Here's how the part is built. I have some questions about the finished solid (model axes, mm). Face numbers are marked on the shaded views. A direction names the side the tool comes from. Round coordinates to 2 decimals unless told otherwise and drop trailing zeros. Loops run counter-clockwise (first coordinate to the right, second up) from the corner with the lowest first, then second, coordinate; pieces in that order, holes last. Notation, with made-up numbers: (25, -30) -> (53, -30) arc R8 cw to (53, -20) -> close; hole circle Ø8 at (39.5, 4). An arc over 180 degrees is marked (long way). One line per item, written item: value. Start each with the question number.
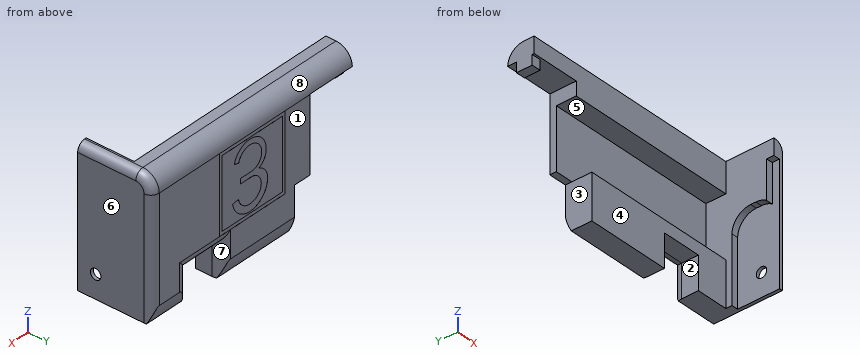
Autodesk Inventor part; units mm, degrees
ref_plane "作業平面1" through (-54.9, 2, -8) normal (1, 0, 0) x (0, 1, 0)
ref_plane "作業平面2" through (-69.8, 2, -8) normal (-1, 0, 0) x (0, 0, 1)
ref_plane "YZ Plane" through (0, 0, 0) normal (1, 0, 0) x (0, 1, 0)
sketch "スケッチ1" plane through (0, 0, 0) normal (1, 0, 0) x (0, 1, 0)
  line L0 (0, 0) -> (22.8, 0)
  line L1 (22.8, 0) -> (22.8, 41.3)
  line L2 (22.8, 41.3) -> (0, 41.3)
  line L3 (0, 41.3) -> (0, 0)
  arc A0 (2, -7.1682) -> (22.8, 4.7165) centre (7.1, 8.05) ccw
  line L4 (22.8, 36.2) -> (22.8, 4.7165)
  line L5 (22.8, 36.2) -> (12.6, 36.2)
  line L6 (12.6, 36.2) -> (12.6, 28.2)
  line L7 (14.2, 28.2) -> (12.6, 28.2)
  line L8 (14.2, 28.2) -> (14.2, 32.2)
  line L9 (14.2, 32.2) -> (20.8, 32.2)
  line L10 (20.8, 32.2) -> (20.8, 8.3)
  line L11 (14.2, 8.3) -> (20.8, 8.3)
  line L12 (14.2, 4.7954) -> (14.2, 8.3)
  line L13 (14.2, 0) -> (14.2, 4.7954)
  line L14 (2, 0) -> (14.2, 0)
  line L15 (2, 0) -> (2, -7.1682)
  line L16 (12.6, 42.3) -> (14.6, 42.3)
  dimension "d2" = 1
extrude "押し出し1" add sketch "スケッチ1" along normal blind 1 contours L3 L2 L1 L5 L6 L7 L8 L9 L10 L11 L12 L13 L0 | L13 L12 L11 L10 L9 L8 L7 L6 L5 L1 A0 L0 | A0 L1 L0
sketch "スケッチ2" plane through (0, 0, 0) normal (-1, 0, 0) x (0, 0, 1)
  line L0 (24.3426, 2) -> (36.2, 2)
  line L1 (36.2, 0) -> (36.2, 2)
  arc A0 (25.6, 7.1) -> (20.1, 12.6) centre (20.1, 7.1) ccw
  line L2 (25.6, 7.1) -> (25.6, 5.5)
  arc A1 (24.3426, 2) -> (25.6, 5.5) centre (20.1, 5.5) ccw
  line L3 (0, 12.6) -> (20.1, 12.6)
  line L4 (0, 22.8) -> (41.3, 22.8)
  line L5 (0, 0) -> (0, 22.8)
  line L6 (41.3, 0) -> (0, 0)
  line L7 (41.3, 22.8) -> (41.3, 0)
  line L8 (0, 12.8) -> (20.1, 12.8)
  arc A2 (25.8, 7.1) -> (20.1, 12.8) centre (20.1, 7.1) ccw
  arc A3 (24.7476, 2.2) -> (25.8, 5.5) centre (20.1, 5.5) ccw
  line L9 (25.8, 5.5) -> (25.8, 7.1)
  line L10 (24.7476, 2.2) -> (36.4, 2.2)
  line L11 (36.4, 2.2) -> (36.4, 0)
  line L12 (41.3, 0) -> (0, 0)
  line L13 (0, 0) -> (0, 22.8)
extrude "押し出し2" add sketch "スケッチ2" along normal blind 2 contours L11 L10 A3 L9 A2 L8 L5 L4 L7 L6
sketch "スケッチ3" plane through (-2, 0, 0) normal (-1, 0, 0) x (0, 0, 1)
  line L0 (28.2, 12.6) -> (50.1, 12.6)
  line L1 (0, 14.2) -> (4.55, 14.2)
  line L2 (41.3, 0) -> (41.3, 22.8)
  line L3 (41.3, 22.8) -> (0, 22.8)
  line L4 (0, 22.8) -> (0, 12.8)
  line L5 (0, 12.8) -> (20.1, 12.8)
  arc A0 (25.8, 7.1) -> (20.1, 12.8) centre (20.1, 7.1) ccw
  line L6 (25.8, 7.1) -> (25.8, 5.5)
  arc A1 (24.7476, 2.2) -> (25.8, 5.5) centre (20.1, 5.5) ccw
  line L7 (24.7476, 2.2) -> (36.4, 2.2)
  line L8 (36.4, 2.2) -> (36.4, 0)
  line L9 (36.4, 0) -> (41.3, 0)
  line L10 (41.3, 0) -> (41.3, 22.8)
  line L11 (0, 14.7) -> (41.3, 14.7)
  point P0 (0, 0)
  dimension "d9" = 0.5
extrude "押し出し3" add sketch "スケッチ3" along normal blind 47.4 contours L11 L4 L3 L2
sketch "スケッチ4" plane through (-49.4, 0, 0) normal (-1, 0, 0) x (0, 0, 1)
  line L0 (11.075, 12.3395) -> (13.693, 16.874)
  line L1 (13.693, 16.874) -> (13.693, 22.8)
  line L2 (41.3, 22.8) -> (0, 22.8)
  line L3 (0, 22.8) -> (0, 14.7)
  line L4 (0, 14.7) -> (41.3, 14.7)
  line L5 (41.3, 14.7) -> (41.3, 22.8)
  line L6 (41.3, 22.8) -> (0, 22.8)
  arc A0 (4.7165, 22.8) -> (-7.1682, 2) centre (8.05, 7.1) ccw
  line L7 (36.2, 22.8) -> (4.7165, 22.8)
  line L8 (36.2, 22.8) -> (36.2, 12.6)
  line L9 (36.2, 12.6) -> (28.2, 12.6)
  line L10 (28.2, 14.2) -> (28.2, 12.6)
  line L11 (28.2, 14.2) -> (32.2, 14.2)
  line L12 (32.2, 14.2) -> (32.2, 20.8)
  line L13 (32.2, 20.8) -> (8.3, 20.8)
  line L14 (8.3, 14.2) -> (8.3, 20.8)
  line L15 (4.7954, 14.2) -> (8.3, 14.2)
  line L16 (0, 14.2) -> (4.7954, 14.2)
  line L17 (0, 2) -> (0, 14.2)
  line L18 (0, 2) -> (-7.1682, 2)
  point P0 (0, 0)
  point P1 (13.693, 20.8)
  point P2 (32.2, 14.7)
ref_plane "作業平面1" through (-54.9, 2, -8) normal (1, 0, 0) x (0, 1, 0)
extrude "押し出し4" add sketch "スケッチ4" along normal up to surface (5.5 mm away) contours L12 L13 L1 L2 L8 L4 | L8 L2 L5 L4
sketch "スケッチ5" plane through (-54.9, 14.7, 41.3) normal (-1, 0, 0) x (0, 0, 1)
  line L0 (-27.607, 6.1) -> (-9.1, 6.1)
  line L1 (-9.1, 6.1) -> (-9.1, 0)
  line L2 (-9.1, 0) -> (0, 0)
  line L3 (0, 0) -> (0, 8.1)
  line L4 (0, 8.1) -> (-27.607, 8.1)
  line L5 (-27.607, 8.1) -> (-27.607, 6.1)
  line L6 (-5.1, -12.7) -> (-5.1, 0.5)
  line L7 (0, 0) -> (-41.3, 0)
  line L8 (-4.9, 0) -> (-4.9, 8.1)
  point P0 (-41.3, -14.7)
  point P1 (-4.9, 0)
  dimension "d14" = 0.2
ref_plane "作業平面2" through (-69.8, 2, -8) normal (-1, 0, 0) x (0, 0, 1)
extrude "押し出し5" add sketch "スケッチ5" along normal up to surface (14.9 mm away) contours L4 L3 L2 L8
sketch "スケッチ6" plane through (-49.4, 0, 0) normal (-1, 0, 0) x (0, 0, 1)
  line L0 (13.693, 20.8) -> (13.693, 22.8)
  line L1 (13.693, 22.8) -> (0, 22.8)
  line L2 (0, 22.8) -> (0, 14.7)
  line L3 (0, 14.7) -> (32.2, 14.7)
  line L4 (32.2, 14.7) -> (32.2, 20.8)
  line L5 (32.2, 20.8) -> (13.693, 20.8)
  line L6 (13.693, 20.8) -> (13.693, 14.7)
  point P0 (0, 0)
extrude "押し出し6" cut sketch "スケッチ6" against normal up to surface (47.4 mm away) contours L5 L4 L3 L6
fillet "フィレット1" radius 5 1 edges at (-34.4, 22.8, 41.3)
fillet "フィレット2" radius 2.5 3 edges at (1, 22.8, 18.15) (1, 21.3355, 39.8355) (1, 8.9, 41.3)
sketch "スケッチ7" plane through (-49.4, 0, 0) normal (-1, 0, 0) x (0, 0, 1)
  arc A0 (4.7165, 22.8) -> (-7.1682, 2) centre (8.05, 7.1) ccw
  line L0 (13.693, 22.8) -> (0, 22.8)
  arc A1 (4.7165, 22.8) -> (-7.1682, 2) centre (8.05, 7.1) ccw
  line L1 (0, 22.8) -> (0, 14.7)
  point P0 (0, 0)
  point P1 (0, 20.9852)
extrude "押し出し7" cut sketch "スケッチ7" against normal through all
sketch "スケッチ8" plane through (0, 0, 0) normal (0, 0, -1) x (-1, 0, 0)
  line L0 (23.7, 13.1) -> (23.7, 1.1)
  line L1 (2, 14.7) -> (49.4, 14.7)
  line L2 (1.5, 22.8) -> (49.4, 22.8)
  line L3 (2, 14.7) -> (69.8, 14.7)
  line L4 (23.7, 14.7) -> (11.7, 14.7)
  line L5 (11.7, 14.7) -> (11.7, 22.8)
  line L6 (11.7, 22.8) -> (23.7, 22.8)
  line L7 (23.7, 22.8) -> (23.7, 14.7)
  point P0 (0, 0)
  point P1 (11.7, 14.7)
  dimension "d23" = 12
extrude "押し出し8" cut sketch "スケッチ8" against normal blind 10
fillet "フィレット3" radius 3 3 edges at (-23.7, 22.8, 7.3582) (-11.7, 22.8, 7.3582) (-17.7, 22.8, 10)
sketch "スケッチ9" plane through (-69.8, 14.7, 36.4) normal (-1, 0, 0) x (0, 0, 1)
  line L0 (-0.2, 0.5) -> (-3.2, 0.5)
  line L1 (-0.2, 5.5) -> (-0.2, 0.5)
  line L2 (-3.2, 5.5) -> (-0.2, 5.5)
  line L3 (-3.2, 0.5) -> (-3.2, 5.5)
  line L4 (-3, 5.4) -> (0, 5.4)
  line L5 (0, 5.4) -> (0, 0.6)
  line L6 (0, 0.6) -> (-3, 0.6)
  line L7 (-3, 0.6) -> (-3, 5.4)
  arc A0 (4.9, 3.1) -> (0, 8.099) centre (-0.1, 3.1) ccw
  line L8 (0, 0) -> (0, 8.099)
  line L9 (4.9, 0) -> (0, 0)
  line L10 (4.9, 3.1) -> (4.9, 0)
  line L11 (0, 0) -> (0, 8.099)
  point P0 (-36.4, -14.7)
  point P1 (-0.2, 3)
  point P2 (-3, 3)
  dimension "d27" = 4.8
extrude "押し出し9" add sketch "スケッチ9" against normal blind 2.8 contours L6 L7 L4 L1 | L1 L4 L5 L6
sketch "スケッチ10" plane through (1, 0, 0) normal (1, 0, 0) x (0, 0, -1)
  circle A0 centre (-7.05, 5.504) radius 1.6
  arc A1 (-4.65, 5.508) -> (-6.95, 8) centre (-7.15, 5.508) ccw
  arc A2 (-6.95, 8) -> (-9.45, 5.5) centre (-6.95, 5.5) ccw
  line L0 (-7.15, 5.508) -> (-6.95, 5.5)
  point P0 (0, 0)
  dimension "d30" = 3.2
extrude "押し出し10" cut sketch "スケッチ10" against normal through all
sketch "スケッチ11" plane through (-54.9, 22.8, 13.693) normal (0, 1, 0) x (1, 0, 0)
  line L0 (53.4, -22.607) -> (0, -22.607)
  line L1 (32.15, -22.607) -> (8.85, -22.607)
  line L2 (8.85, -22.607) -> (8.85, 0.693)
  line L3 (8.85, 0.693) -> (32.15, 0.693)
  line L4 (32.15, 0.693) -> (32.15, -22.607)
  line L5 (28.2, 0.693) -> (46.2, 0.693)
  line L6 (20.5, -22.607) -> (20.5, -17.7274)
  line L7 (55.9, -22.607) -> (55.9, 13.693)
  line L8 (-14.9, -27.607) -> (-14.9, -22.707)
  line L9 (55.9, -22.607) -> (55.9, 7.9184)
  line L10 (-14.9, -27.607) -> (-14.9, -22.707)
  line L11 (-14.9, -27.607) -> (-14.9, -22.707)
  line L12 (10.35, -0.807) -> (30.65, -0.807)
  line L13 (30.65, -0.807) -> (30.65, -21.107)
  line L14 (30.65, -21.107) -> (10.35, -21.107)
  line L15 (10.35, -21.107) -> (10.35, -0.807)
  line L16 (9.85, -0.307) -> (31.15, -0.307)
  line L17 (31.15, -0.307) -> (31.15, -21.607)
  line L18 (31.15, -21.607) -> (9.85, -21.607)
  line L19 (9.85, -21.607) -> (9.85, -0.307)
  line L20 (-14.2639, 8.2606) -> (-10.5139, 8.2606)
  circle A0 centre (21.3, -7.057) radius 6.25
  circle A1 centre (21.3, -15.357) radius 5.75
  circle A2 centre (21.3, -7.057) radius 4.15
  circle A3 centre (21.3, -15.357) radius 4.15
  line L21 (24.6204, -10.2528) -> (18.6525, -10.2528)
  line L22 (18.6525, -10.2528) -> (18.6525, -11.7867)
  line L23 (18.6525, -11.7867) -> (24.6204, -11.7867)
  line L24 (24.6204, -11.7867) -> (24.6204, -10.2528)
  arc A4 (15.053, -6.8649) -> (21.3, -11.207) centre (19.5885, -7.0044) ccw
  arc A5 (21.3, -11.207) -> (15.55, -15.3584) centre (19.9229, -15.3573) ccw
  arc A6 (20.7203, -11.7867) -> (17.15, -15.357) centre (20.7203, -15.357) ccw
  arc A7 (18.3285, -4.16) -> (20.8976, -10.2528) centre (20.8976, -6.6647) ccw
  line L25 (21.3, -15.357) -> (26.8541, -16.8452)
  line L26 (21.3, -7.057) -> (27.455, -5.9717)
  point P0 (54.9, 13.693)
  point P1 (20.5, 14.3955)
  point P2 (30.65, -10.957)
  point P3 (31.15, -10.957)
  point P4 (20.5, -0.807)
  point P5 (20.5, -0.307)
  point P6 (20.5, 3.8955)
  point P7 (18.6525, -11.0197)
  point P8 (32.15, -10.957)
  point P9 (20.5, -21.607)
  point P10 (25.387, -6.3363)
  point P11 (18.2184, -11.3303)
  point P12 (25.3086, -16.4311)
  point P13 (8.85, -22.607)
  dimension "d33" = 35.4
  dimension "d34" = 35.4
  dimension "d35" = 23.3
  dimension "d36" = 23.3
  dimension "d40" = 0.5
  dimension "d49" = 1
  dimension "d51" = 11.5
  dimension "d52" = 12.5
  dimension "d53" = 0.8
  dimension "d54" = 80
  dimension "d55" = 75
extrude "押し出し11" cut sketch "スケッチ11" against normal blind 0.01 contours L0 L2 L3 L4 | A1 A5 A0 A3 L6 | L6 A3 L25 A1 | A3 A0 A6 | A5 A4 L22 L23 A3 A0 | A0 L26 A2 A1 A4 | A3 L23 A6 A0 | A1 L22 A5 A4 | A5 L22 A4 | L23 L22 A4 A3 | A3 A4 L23 | A2 A7 A1 | L21 A2 A5 | A1 A7 L21 | A2 A5 L22 | L22 A5 A2 A3 A4 | L24 L23 A3 A2 A1 | A1 L21 L24 | A3 A4 | A5 A2 picked at (17.7249, -13.3851) picked at (19.4043, -11.9435) picked at (18.4353, -9.7598) picked at (19.6416, -10.192)
equation "\"d33\" = d34"
equation "\"d36\" = d35"
equation "\"d4\" = d3"
equation "\"d5\" = d4"
equation "\"d6\" = d5"
properties part number "hand_finger_cover_3"
Q1. I want a section at D-D on x = -16. Please give me the cut outline in (y, z), plus the area to 3 significant figures.
Q2. I want a section at A-A on z = 7.05. Please give me the cut outline in (x, y).
Q3. Which directions (+Z, -Z, +X, -X, +Y, -Y) give clear straight access to the entire face, cutting with the end or side of a thin tool? Please do the marked faces 1, 2, 3, 4 and 5.
Q4. I want a section at B-B on x = -5.5. Please give me the cut outline in (y, z), plus the area to 3 significant figures.
Q5. If we mould it in two halves opening along X, with no side actions, what happens to the marked faces 6, 7 and 8? For each: released by +X, released by -X, zero draft, split by the parting line, or undercut.
Q6. Will these pins go through, and if not, where does the flat tip stop? P1, Ø2.5, axis at y = 5.504, z = 7.05, coming from the -X side; P2, Ø2, axis at x = -68, y = 18, coming from the -Z side; P3, Ø5, axis at x = -50, z = 23.5, coming from the -Y side; P4, Ø4, axis at x = -16, y = 18.5, coming from the -Z side.
Q7. If I drill on line 1 along Z through (x, y) = (-36, 16); line 2 along Y through (x, z) = (-48, 36.5); line 3 along X through (y, z) = (18.25, 7), over which ranges is the centre line in solid material (lowest first)?
Answers below:
1. outline: (14.7, 10) -> (19.8, 10) arc R3 ccw to (22.8, 13) -> (22.8, 36.3) arc R5 ccw to (17.8, 41.3) -> (14.7, 41.3) -> (14.7, 32.2) -> (20.8, 32.2) -> (20.8, 13.69) -> (14.7, 13.69) -> close
1. area: 133 mm^2
2. outline: (-49.4, 14.7) -> (-23.7, 14.7) -> (-23.7, 19.8) arc R3 ccw to (-26.7, 22.8) -> (-49.4, 22.8) -> close; (-11.7, 14.7) -> (-2, 14.7) -> (-2, 12.8) -> (0, 12.8) -> (0, 7.1) -> (1, 7.1) -> (1, 20.3) arc R2.5 ccw to (-1.5, 22.8) -> (-8.7, 22.8) arc R3 ccw to (-11.7, 19.8) -> close; (0, 0) -> (1, 0) -> (1, 3.9) -> (0, 3.9) -> close
3. face 1: +Z, -Z, +X, -X, +Y
3. face 2: -Z, +Y, -Y
3. face 3: -Z, -X, +Y, -Y
3. face 4: +Z, -Z, -X, -Y
3. face 5: -X, -Y
4. outline: (14.7, 0) -> (20.99, 0) arc R16.05 ccw to (22.8, 4.72) -> (22.8, 36.3) arc R5 ccw to (17.8, 41.3) -> (14.7, 41.3) -> (14.7, 32.2) -> (20.8, 32.2) -> (20.8, 13.69) -> (14.7, 13.69) -> close
4. area: 213 mm^2
5. face 6: released by +X
5. face 7: undercut
5. face 8: zero draft
6. P1: passes through
6. P2: stops at z = 33.4
6. P3: stops at y = 20.8
6. P4: stops at z = 10
7. line 1: z = 0 to 13.69, 32.2 to 41.3
7. line 2: y = 14.7 to 22.8
7. line 3: x = -49.4 to -23.7, -11.7 to 1
